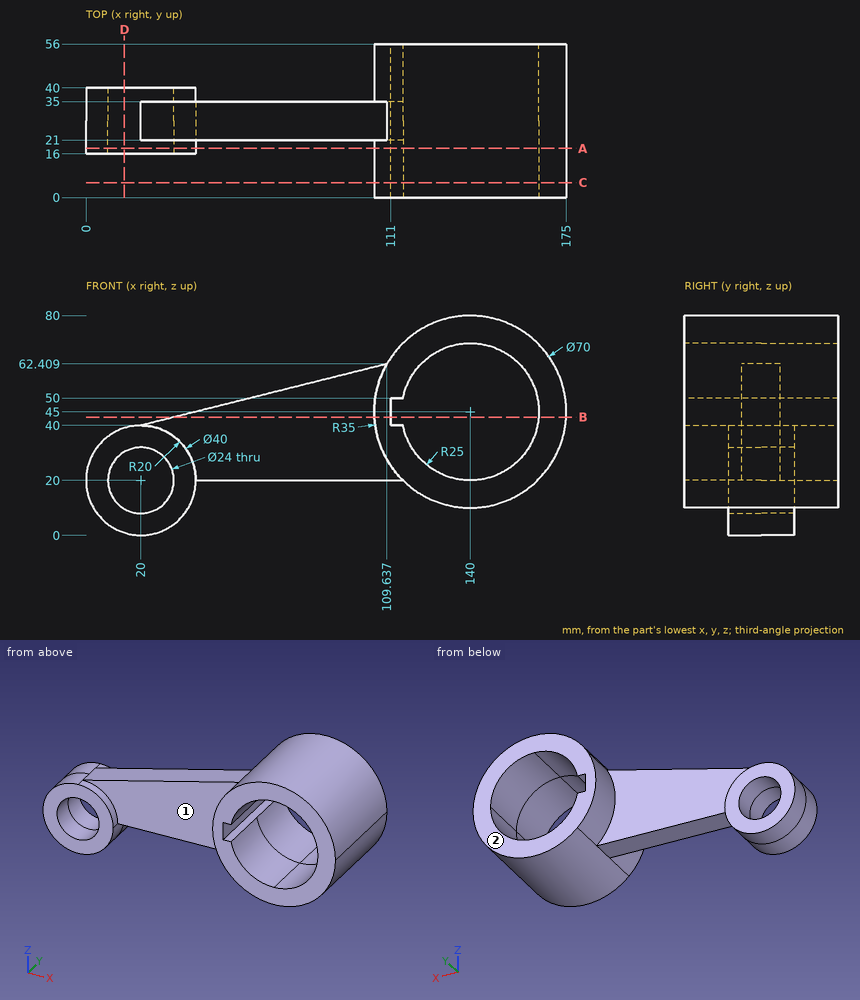
Input: dimensioned drawing with shaded views. Units: mm. Origin: part minimum x, y, z. Give positions to 0.01 mm unless a question says otherwise; leave off trailing zeros. Loops run counter-clockwise (first coordinate to the right, second up) from the corner with the lowest first, then second, coordinate; pieces in that order, holes last. Notation, with made-up numbers: M 15,5 L 57,5 A29 cw 57,30 Z; hole C 84.5,19 d10. An arc over 180 degrees is marked long. Put each result on its own line as item: value. Start each with the question number.
1) Ray query, line 1 along X through (y, z) = (17, 29); line 2 along X through (y, z) = (34, 31) (1 decimal); line 3 along Y through (x, z) = (47.5, 37). Return the intervals inside material, ascending.
2) Cut plane C-C (y = 5.5). Output: boundary loops of the cut face in (x, z) (1 decimal).
3) Contact query for flat-ended pins moving along their axis: pin 1 (1.4 mm diameter, centred on x = 112.5, y = 20.5, fed in from +Z); pin 2 (5 mm diameter, centred on y = 42, z = 34, fed in from +X); pin 3 (15.5 mm diameter, centred on x = 63.5, y = 29, fed in from -Z); pin 4 (21.5 mm diameter, centred on x = 20, z = 20, fed in from -Y). Output: stop coordinate, or through.
4) Pull-direction query (X, two-part tool) for the marked faces 1 and 2; classes: pulls with the +X half, pulls with the -X half, needs draft (parallel to the pull), parting line crosses it, or undercut.
5) Cut plane A-A (y = 18). Output: boundary loops of the cut face in (x, z) (1 decimal), then the cut area to 3 significant figures.
6) Cut plane D-D (x = 14). Output: boundary loops of the cut face in (y, z).
7) Cut plane B-B (z = 43). Output: boundary loops of the cut face in (x, y).
Verdict:
1. line 1: 2.14 to 12.06, 27.94 to 37.86, 108.87 to 120.79, 159.21 to 171.13
1. line 2: 3.3 to 15.2, 24.8 to 119.3, 160.7 to 172.1
1. line 3: 21 to 35
2. outline: C 140,45 d70; hole M 111,40 L 115.5,40 A25 ccw long 115.5,50 L 111,50 Z
3. pin 1: z = 67.51
3. pin 2: x = 173.95
3. pin 3: z = 20
3. pin 4: through
4. face 1: undercut
4. face 2: needs draft
5. outline: C 20,20 d40; C 140,45 d70; hole C 20,20 d24; hole M 111,40 L 115.5,40 A25 ccw long 115.5,50 L 111,50 Z
5. area: 2,650 mm2
6. outline: M 16,0.92 L 40,0.92 L 40,9.61 L 16,9.61 Z; M 16,30.39 L 40,30.39 L 40,39.08 L 16,39.08 Z
7. outline: M 32,21 L 105.06,21 L 105.06,0 L 111,0 L 111,56 L 105.06,56 L 105.06,35 L 32,35 Z; M 164.92,0 L 174.94,0 L 174.94,56 L 164.92,56 Z
